```python
from build123d import *

# Parameters (mm, degrees)
SALIENTE_EXTRUIR1_DEPTH = 14
CORTAR_EXTRUIR1_DEPTH   = 11
CORTAR_EXTRUIR2_DEPTH   = 8
CROQUIS4_OUTSIDE_W      = 214.456
CROQUIS4_OUTSIDE_H      = 206.311
CORTAR_EXTRUIR4_DEPTH   = 2
CROQUIS6_R              = 1.25
CORTAR_EXTRUIR6_DEPTH   = 7


with BuildPart() as part:
    # Croquis1 → Saliente-Extruir1 (new body)
    with BuildSketch(Plane(origin=(0, 0, 0), x_dir=(1, 0, 0), z_dir=(0, 1, 0))):
        Polygon((0, 87.5), (-19.644973975, 27.038987008), (-83.217445176, 27.038987008), (-31.7862356, -10.327974016), (-51.431209576, -70.788987008), (0, -33.422025984), (51.431209576, -70.788987008), (31.7862356, -10.327974016), (83.217445176, 27.038987008), (19.644973975, 27.038987008), align=None)
    extrude(amount=SALIENTE_EXTRUIR1_DEPTH)

    # Croquis2 → Cortar-Extruir1 (cut)
    with BuildSketch(Plane(origin=(0, 14, 0), x_dir=(1, 0, 0), z_dir=(0, 1, 0))):
        Polygon((31.866240983, -53.484035323), (41.019130301, -46.83407198), (28.847309339, -9.373058987), (60.713550322, 13.779120295), (57.217457698, 24.538987008), (17.828617655, 24.538987008), (5.656796693, 62), (-5.656796693, 62), (-17.828617655, 24.538987008), (-57.217457698, 24.538987008), (-60.713550322, 13.779120295), (-28.847309339, -9.373058987), (-41.019130301, -46.83407198), (-31.866240983, -53.484035323), (0, -30.331856041), align=None)
    extrude(amount=-CORTAR_EXTRUIR1_DEPTH, mode=Mode.SUBTRACT)

    # Croquis3 → Cortar-Extruir2 (cut)
    with BuildSketch(Plane(origin=(0, 14, 0), x_dir=(1, 0, 0), z_dir=(0, 1, 0))):
        Polygon((57.944000226, 25.538987008), (18.555160183, 25.538987008), (6.383339221, 63), (-6.383339221, 63), (-18.555160183, 25.538987008), (-57.944000226, 25.538987008), (-61.889120827, 13.397154283), (-30.022879843, -9.755024999), (-42.194700805, -47.216037991), (-31.866240983, -54.7201033), (0, -31.567924018), (31.866240983, -54.7201033), (42.194700805, -47.216037991), (30.022879843, -9.755024999), (61.889120827, 13.397154283), align=None)
        Polygon((57.217457698, 24.538987008), (17.828617655, 24.538987008), (5.656796693, 62), (-5.656796693, 62), (-17.828617655, 24.538987008), (-57.217457698, 24.538987008), (-60.713550322, 13.779120295), (-28.847309339, -9.373058987), (-41.019130301, -46.83407198), (-31.866240983, -53.484035323), (0, -30.331856041), (31.866240983, -53.484035323), (41.019130301, -46.83407198), (28.847309339, -9.373058987), (60.713550322, 13.779120295), align=None, mode=Mode.SUBTRACT)
    extrude(amount=-CORTAR_EXTRUIR2_DEPTH, mode=Mode.SUBTRACT)

    # Croquis4 outside → Cortar-Extruir4 (cut)
    with BuildSketch(Plane(origin=(0, 14, 0), x_dir=(1, 0, 0), z_dir=(0, 1, 0))):
        with Locations((0, 8.3555)):
            Rectangle(CROQUIS4_OUTSIDE_W, CROQUIS4_OUTSIDE_H)
        Polygon((19.644973975, 27.038987008), (0, 87.5), (-19.644973975, 27.038987008), (-83.217445176, 27.038987008), (-31.7862356, -10.327974016), (-51.431209576, -70.788987008), (0, -33.422025984), (51.431209576, -70.788987008), (31.7862356, -10.327974016), (83.217445176, 27.038987008), align=None, mode=Mode.SUBTRACT)
        Polygon((18.918431447, 26.038987008), (0, 84.263932023), (-18.918431447, 26.038987008), (-80.139761639, 26.038987008), (-30.610665096, -9.946008004), (-49.529096543, -68.170953019), (0, -32.185958007), (49.529096543, -68.170953019), (30.610665096, -9.946008004), (80.139761639, 26.038987008), align=None)
    extrude(amount=-CORTAR_EXTRUIR4_DEPTH, mode=Mode.SUBTRACT)

    # Croquis6 → Cortar-Extruir6 (cut)
    with BuildSketch(Plane(origin=(0, 12, 0), x_dir=(1, 0, 0), z_dir=(0, 1, 0))):
        with Locations((-67.049484399, 21.785698103)):
            Circle(CROQUIS6_R)
        with Locations((0, 70.5)):
            Circle(CROQUIS6_R)
        with Locations((67.049484399, 21.785698103)):
            Circle(CROQUIS6_R)
        with Locations((41.438860287, -57.035698103)):
            Circle(CROQUIS6_R)
        with Locations((-41.438860287, -57.035698103)):
            Circle(CROQUIS6_R)
    extrude(amount=-CORTAR_EXTRUIR6_DEPTH, mode=Mode.SUBTRACT)


solid = part.part
```
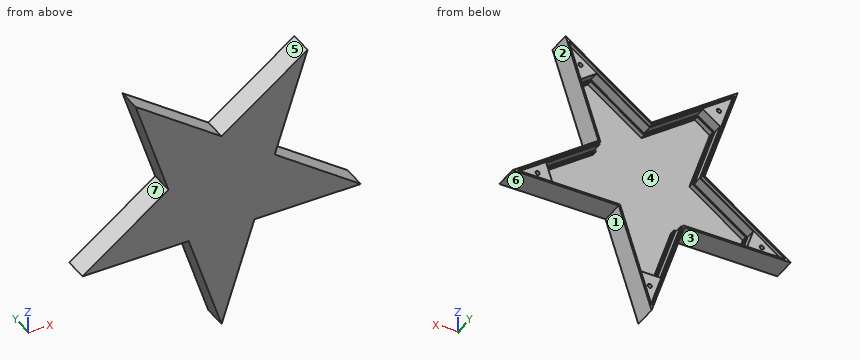
Input: part model. Units: mm. Frame: model coordinates. Face numbers are marked on the shaded views. A direction names the side the tool comes from. Give positions to 0.01 mm unless a question says otherwise; leave off trailing zeros. Order: outer loops, then holes, each group sorted by start corner. A loop starts at its lowest first (then second) coordinate and runs counter-clockwise, first axis right, second up. Notation, with made-up numbers: M 54,25 L 84,25 A24 ccw 84,45 Z; hole C 41,-5 d2. An arc over 180 degrees is marked long. Return JSON: item names as keys, results as strings.
Item 1: Access query for the marked faces 1, 2 and 3. Directions: +Z, -Z, +X, -X, +Y, -Y. A direction counts if a zero-diameter tool reaches every point of the face in a straight line with its end or side. Return the directions, or none.
Solutions:
{"face 1": "-Z, +X, +Y, -Y", "face 2": "+X, +Y, -Y", "face 3": "-Z, -X, +Y, -Y"}
Item 2: Pull-direction query (Z, two-part tool) for the marked faces 4, 5, 6 and 7; classes: +Z half, -Z half, draft (parallel to the pull), parting line (faces both ways), or undercut.
Solutions:
{"face 4": "undercut", "face 5": "+Z half", "face 6": "-Z half", "face 7": "undercut"}
Item 3: Cut plane C-C (z = -67). Return loops of the section in (x, y).
Solutions:
{"outline": "M -6.66,0 L 6.66,0 L 6.66,14 L 5.61,14 L 5.61,12 L -5.61,12 L -5.61,14 L -6.66,14 Z"}
Item 4: First-contact query: P1, Ø3, axis at x = 41, y = 8.5, coming from the +Z side; P2, Ø2, axis at x = -61.5, y = 10.5, coming from the -Z side; P3, Ø1.5, axis at x = 67.05, z = -21.79, coming from the -Y side; P4, Ø3.5, axis at x = -34, y = 5, coming from the +Z side. Flat tips, straight axial feed; report the tip coordinate or a pass-through.
Solutions:
{"P1": "z = 64.3", "P2": "z = -27.04", "P3": "y = 0", "P4": "z = 59.4"}
Item 5: Cut plane D-D (z = 4). Return loops of the section in (x, y), then the cut area to 3 significant figures.
Solutions:
{"outline": "M -40.5,0 L 40.5,0 L 40.5,14 L 38.79,14 L 38.79,12 L 37.94,12 L 37.94,6 L 36.24,6 L 36.24,3 L -36.24,3 L -36.24,6 L -37.94,6 L -37.94,12 L -38.79,12 L -38.79,14 L -40.5,14 Z", "area": "306 mm^2"}
Item 6: Cut plane B-B (y = 10). State how many separate pieces and enclosed holes the cut face has, then the cut area to 3 significant figures.
Solutions:
{"separate pieces": "1", "enclosed holes": "6", "area": "1,530 mm^2"}
Item 7: Ray query, probe 1 along X at (y, z) = (3.25, 40.5); probe 2 along X at (y, z) = (5, 62); probe 3 along X at (y, z) = (8.5, 3). Return the intervals inside material, ascending.
Solutions:
{"probe 1": "-41.59 to -38.96, -14 to -9.74, 9.74 to 14, 38.96 to 41.59", "probe 2": "-48.58 to -39.33, 39.33 to 48.58", "probe 3": "-41.87 to -39.32, 39.32 to 41.87"}
Item 8: Cut plane A-A (z = -29). Return loops of the section in (x, y), then the cut area to 3 significant figures.
Solutions:
{"outline": "M -19.01,0 L 19.01,0 L 19.01,14 L 17.96,14 L 17.96,12 L 17.43,12 L 17.43,6 L 16.38,6 L 16.38,3 L -16.38,3 L -16.38,6 L -17.43,6 L -17.43,12 L -17.96,12 L -17.96,14 L -19.01,14 Z", "area": "153 mm^2"}
